Design review of the part built by this model. Coordinates are the model's own, in mm. A direction names the side the tool comes from. Give positions to 0.01 mm unless a question says otherwise; leave off trailing zeros. Order: outer loops, then holes, each group sorted by start corner. A loop starts at its lowest first (then second) coordinate and runs counter-clockwise, first axis right, second up. Notation, with made-up numbers: (-36, 79) - (8, 79) arc R15 ccw to (8, 98) - close; hole circle Ø7 at (1, 12.25). An arc over 180 degrees is marked (long way). Write each question's results on one line, items separated by ' | '. Start each with the question number.
Autodesk Inventor part; units mm, degrees
ref_plane "YZ Plane" through (0, 0, 0) normal (1, 0, 0) x (0, 1, 0)
ref_plane "XZ Plane" through (0, 0, 0) normal (0, 1, 0) x (-1, 0, 0)
ref_plane "XY Plane" through (0, 0, 0) normal (0, 0, 1) x (1, 0, 0)
sketch "Sketch1" plane through (0, 0, 0) normal (0, 0, 1) x (1, 0, 0)
  line L0 (27.09, -10) -> (-27.09, -10)
  line L1 (-27.09, -10) -> (-27.09, 10)
  line L2 (-27.09, 10) -> (27.09, 10)
  line L3 (27.09, 10) -> (27.09, -10)
  line L4 (27.09, -10) -> (-27.09, 10) construction
  line L5 (-27.09, -10) -> (27.09, 10) construction
  point P0 (0, 0)
  dimension "d0" = 54.18
  dimension "d1" = 20
extrude "Plate1" add sketch "Sketch1" along normal blind 1.5
sketch "Sketch2" plane through (-25.59, 10, 1.5) normal (-1, 0, 0) x (0, -1, 0)
  line L0 (20, 0) -> (0, 0)
  line L1 (0, 0) -> (0, -22)
  line L2 (0, -22) -> (20, -22)
  line L3 (20, -22) -> (20, 0)
edge flange "Flange1" height 22 angle 90 thickness 1.5 bend radius 0.31 thickness toward (-1, 0, 0) relief tear relief width 1.5 relief depth 0.75 corner gap 0.31 corner form 0 edges at (-27.09, 0, 0) (27.09, 0, 0) wall of the first edge with corners at (-25.59, -10, 1.5) (-25.59, 10, 1.5) (-25.59, 10, -20.5) (-25.59, -10, -20.5)
bend "Bend1"
corner "Corner1"
sketch "Sketch3" plane through (27.09, -10, -20.5) normal (1, 0, 0) x (0, 0, -1)
  line L0 (-20.19, 20) -> (-20.19, 0) construction
  line L1 (0, 0) -> (-20.19, 0) construction
  line L2 (0, 20) -> (0, 0) construction
  line L3 (-20.19, 20) -> (0, 20) construction
  line L4 (0, 20) -> (-20.19, 0) construction
  line L5 (0, 0) -> (-20.19, 20) construction
  point P0 (-20.5, 10)
  point P1 (-16.095, 15.9435)
  point P2 (-4.095, 15.9435)
  point P3 (-16.095, 4.0565)
  point P4 (-4.095, 4.0565)
  dimension "d13" = 12
hole "Hole1" at (27.09, 5.9435, -4.405) at (27.09, 5.9435, -16.405) at (27.09, -5.9435, -4.405) at (27.09, -5.9435, -16.405) direction (-1, 0, 0) diameter 1.567 end through all
equation "\"d2\" = Thickness"
equation "\"d3\" = BendReliefWidth"
equation "\"d4\" = BendReliefDepth"
equation "\"d5\" = MinimumRemnant"
equation "\"d6\" = TransitionRadius"
equation "\"d9\" = BendRadius"
equation "\"d10\" = CornerReliefSize"
equation "\"d11\" = GapSize"
equation "\"d12\" = JacobiRadiusSize"
equation "\"BendReliefWidth\" = Thickness"
equation "\"BendReliefDepth\" = 0.5 * Thickness"
equation "\"CornerReliefSize\" = 4 * Thickness"
equation "\"MinimumRemnant\" = 2 * Thickness"
equation "\"TransitionRadius\" = BendRadius"
equation "\"JacobiRadiusSize\" = BendRadius"
equation "\"GapSize\" = Thickness"
properties part number "axis_3_bottom_frame(middle)" material "Aluminum 6061-AHC"
Q1. Machinability: for faces 4 (the cylindrical face through (26.33, -5.978, -15.622)), 5 (the flat face through (-25.59, 0, -10)), which of the approach directions +Z, -Z, +X, -X, +Y, -Y give a long, thin tool a straight path to every point of the face, cutting with its end or side? Answer none if there is none.
Q2. Add section C-C (x = -3.5). Give the boundary of the cut face in (y, z), plus the area to 3 significant figures.
Q3. Add section A-A (z = -9). Give the boundary of the cut face in (x, y), plus the area to 3 significant figures.
Q4. Draft analysis for pull direction Y (two halves, no side actions). For faces 1 (the flat face through (-26, 0, -20.5)), 2 (the cylindrical face through (26.33, -6.18, -5.15)), 3 (the flat face through (-0.1, -10, 0.2)), state which applies: pulls with the +Y half, pulls with the -Y half, needs draft (parallel to the pull), parting line crosses it, or undercut.
Q5. For line 1 (X direction, y = -3.25, z = -9.25); line 2 (Z direction, x = -24, y = 4.75); line 3 (X direction, y = -3, z = 0.5), list the stretches that pass through material, from the lowest coordinate up. Write a range as [from, to].
Q6. Add section B-B (y = -0.5). Give the boundary of the cut face in (x, z), plus the area to 3 significant figures.
Q7. Insertion check: pin 1 Ø6 at (x, y) = (-11.5, -3.5) entering from -Z. The pin has a flat end and moves straight along its axis. Give the tip position at first contact, or say it passes through.
Verdict:
1) face 4: +X, -X | face 5: -Z, +Y, -Y
2) outline: (-10, 0) - (10, 0) - (10, 1.5) - (-10, 1.5) - close | area: 30.0 mm2
3) outline: (-27.09, -10) - (-25.59, -10) - (-25.59, 10) - (-27.09, 10) - close; (25.59, -10) - (27.09, -10) - (27.09, 10) - (25.59, 10) - close | area: 60.0 mm2
4) face 1: needs draft | face 2: undercut | face 3: pulls with the -Y half
5) line 1: x = [-27.09, -25.59], [25.59, 27.09] | line 2: z = [0, 1.5] | line 3: x = [-26.9, 26.9]
6) outline: (-27.09, -20.5) - (-25.59, -20.5) - (-25.59, -0.31) arc R0.31 cw to (-25.28, 0) - (25.28, 0) arc R0.31 cw to (25.59, -0.31) - (25.59, -20.5) - (27.09, -20.5) - (27.09, -0.31) arc R1.81 ccw to (25.28, 1.5) - (-25.28, 1.5) arc R1.81 ccw to (-27.09, -0.31) - close | area: 141 mm2
7) pin 1: stops at z = 0
